The model under review builds one solid part; all positions refer to its coordinate system, in mm. Face numbers are marked on the shaded views. A direction names the side the tool comes from. Round coordinates to 2 decimals unless told otherwise and drop trailing zeros. Loops run counter-clockwise (first coordinate to the right, second up) from the corner with the lowest first, then second, coordinate; pieces in that order, holes last. Notation, with made-up numbers: (-16.75, 5.5) -> (28.25, 5.5) arc R31 cw to (28.25, 42.5) -> close; hole circle Ø10 at (25, -40). An arc over 180 degrees is marked (long way). Write each question's results on one line, items separated by ' | '. Start each with the question number.
Item 1: We need section D-D (z = -7.25). Give the boundary of the cut face in (x, y).
Item 2: Tool access review of the marked faces 1 and 2: name each direction out of +Z, -Z, +X, -X, +Y, -Y from which nothing blocks a thin tool from reaching the whole face with its end or side.
Item 3: We need section B-B (x = -30). Give the boundary of the cut face in (y, z), and give its area (3 significant figures).
Item 4: For L1, parallel to Y at x = 30, z = 13; L2, parallel to Y at x = 60, z = 4.5; L3, parallel to Y at x = 38, z = 10.25, list the stretches that pass through material, from the lowest coordinate up. Write a range as from..to.
Item 5: We need section C-C (x = 9.5). Give the boundary of the cut face in (y, z).
Item 6: Clearance check with flat-ended pins moving along their axes: pin 1 Ø6 at (y, z) = (0, -4) entering from +X; pin 2 Ø5.5 at (x, y) = (-59, -1) entering from +Z; pin 3 Ø1.5 at (y, z) = (3, -1.5) entering from -X. State where each tip first meets the part, or that it passes through.
Item 7: We need section A-A (z = 8.5). Give the boundary of the cut face in (x, y), and give its area (3 significant figures).
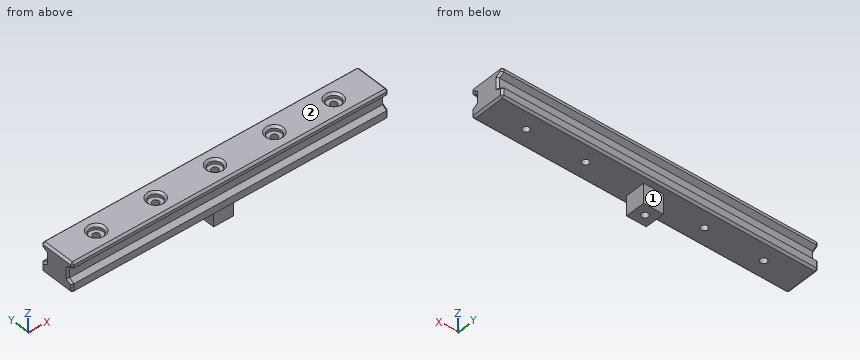
from build123d import *

# Parameters (mm, degrees)
SKETCH1_W                                = 160
SKETCH1_H                                = 18
BOSS_EXTRUDE1_DEPTH                      = 15
CUT_EXTRUDE1_DEPTH                       = 161.953409408
SKETCH3_W                                = 10
SKETCH3_H                                = 10
BOSS_EXTRUDE2_DEPTH                      = 10
CBORE_FOR_M3_PAN_HEAD_SCREW1_D           = 3.4
CBORE_FOR_M3_PAN_HEAD_SCREW1_CBORE_D     = 7
CBORE_FOR_M3_PAN_HEAD_SCREW1_CBORE_DEPTH = 2.4
CHAMFER1_SIZE                            = 1
LPATTERN2_COUNT                          = 3
LPATTERN2_PITCH                          = 30
LPATTERN3_COUNT                          = 3
LPATTERN3_PITCH                          = 30
CHAMFER2_SIZE                            = 1


with BuildPart() as part:
    # Sketch1 → Boss-Extrude1 (new body)
    with BuildSketch(Plane.XY):
        Rectangle(SKETCH1_W, SKETCH1_H)
    extrude(amount=BOSS_EXTRUDE1_DEPTH)

    # Sketch2 → Cut-Extrude1 (cut, through all)
    with BuildSketch(Plane(origin=(80, 0, 0), x_dir=(0, 0, -1), z_dir=(1, 0, 0))):
        Polygon((-12.5, 9), (-4.613248654, 9), (-6.056624327, 6.5), (-11.056624327, 6.5), align=None)
        Polygon((-11.056624327, -6.5), (-12.5, -9), (-4.613248654, -9), (-6.056624327, -6.5), align=None)
    extrude(amount=-CUT_EXTRUDE1_DEPTH, mode=Mode.SUBTRACT)

    # Sketch3 → Boss-Extrude2 (add)
    with BuildSketch(Plane(origin=(0, 0, 0), x_dir=(-1, 0, 0), z_dir=(0, 0, -1))):
        Rectangle(SKETCH3_W, SKETCH3_H)
    extrude(amount=BOSS_EXTRUDE2_DEPTH)

    # CBORE for M3 Pan Head Screw1 (through all)
    with Locations(Plane.XY.offset(15)):
        with Locations((0, 0)):
            cbore_for_m3_pan_head_screw1 = CounterBoreHole(CBORE_FOR_M3_PAN_HEAD_SCREW1_D / 2, CBORE_FOR_M3_PAN_HEAD_SCREW1_CBORE_D / 2, CBORE_FOR_M3_PAN_HEAD_SCREW1_CBORE_DEPTH)

    # Chamfer1
    chamfer1_edges = [part.edges().sort_by_distance(p)[0] for p in [
        (-80, 0, 15),
        (0, -9, 15),
        (80, -9, 2.306624327),
        (-80, -9, 2.306624327),
        (-80, 9, 2.306624327),
        (80, 9, 2.306624327),
        (-80, 7.75, 11.778312164),
        (-80, 7.75, 5.334936491),
        (-80, 6.5, 8.556624327),
        (80, 7.75, 11.778312164),
        (80, 6.5, 8.556624327),
        (80, 7.75, 5.334936491),
        (-80, -6.5, 8.556624327),
        (-80, -7.75, 5.334936491),
        (-80, -7.75, 11.778312164),
        (80, -6.5, 8.556624327),
        (80, -7.75, 11.778312164),
        (80, -7.75, 5.334936491),
        (80, 0, 15),
        (0, -9, 0),
        (-80, 0, 0),
        (0, 9, 0),
        (80, 0, 0),
        (-3.5, 0, 15),
        (0, 9, 15),
        (80, -9, 13.75),
        (-80, -9, 13.75),
        (-80, 9, 13.75),
        (80, 9, 13.75),
    ]]
    chamfer(chamfer1_edges, length=CHAMFER1_SIZE)

    # LPattern2: CBORE for M3 Pan Head Screw1 ×3
    with Locations(*[(i * LPATTERN2_PITCH, 0, 0) for i in range(1, LPATTERN2_COUNT)]):
        add(cbore_for_m3_pan_head_screw1, mode=Mode.SUBTRACT)

    # LPattern3: CBORE for M3 Pan Head Screw1 ×3
    with Locations(*[(-i * LPATTERN3_PITCH, 0, 0) for i in range(1, LPATTERN3_COUNT)]):
        add(cbore_for_m3_pan_head_screw1, mode=Mode.SUBTRACT)

    # Chamfer2
    chamfer2_edges = [part.edges().sort_by_distance(p)[0] for p in [
        (26.5, 0, 15),
        (56.5, 0, 15),
        (-33.5, 0, 15),
        (-63.5, 0, 15),
    ]]
    chamfer(chamfer2_edges, length=CHAMFER2_SIZE)


solid = part.part
Here are the results:
1) outline: (-5, -5) -> (5, -5) -> (5, 5) -> (-5, 5) -> close; hole circle Ø3.4 at (0, 0)
2) face 1: -Z, +X, -X, +Y | face 2: +Z, +X, -X, +Y, -Y
3) outline: (-9, 1) -> (-8, 0) -> (-1.7, 0) -> (-1.7, 12.6) -> (-3.5, 12.6) -> (-3.5, 14) -> (-4.5, 15) -> (-8, 15) -> (-9, 14) -> (-9, 12.5) -> (-6.5, 11.06) -> (-6.5, 6.06) -> (-9, 4.61) -> close; (1.7, 0) -> (8, 0) -> (9, 1) -> (9, 4.61) -> (6.5, 6.06) -> (6.5, 11.06) -> (9, 12.5) -> (9, 14) -> (8, 15) -> (4.5, 15) -> (3.5, 14) -> (3.5, 12.6) -> (1.7, 12.6) -> close | area: 175 mm2
4) L1: y = -9..-3.5, 3.5..9 | L2: y = -9..-1.7, 1.7..9 | L3: y = -6.5..6.5
5) outline: (-9, 1) -> (-8, 0) -> (8, 0) -> (9, 1) -> (9, 4.61) -> (6.5, 6.06) -> (6.5, 11.06) -> (9, 12.5) -> (9, 14) -> (8, 15) -> (-8, 15) -> (-9, 14) -> (-9, 12.5) -> (-6.5, 11.06) -> (-6.5, 6.06) -> (-9, 4.61) -> close
6) pin 1: stops at x = 5 | pin 2: stops at z = 14.66 | pin 3: stops at x = -5
7) outline: (-80, -5.5) -> (-79, -6.5) -> (79, -6.5) -> (80, -5.5) -> (80, 5.5) -> (79, 6.5) -> (-79, 6.5) -> (-80, 5.5) -> close; hole circle Ø3.4 at (-60, 0); hole circle Ø3.4 at (-30, 0); hole circle Ø3.4 at (0, 0); hole circle Ø3.4 at (30, 0); hole circle Ø3.4 at (60, 0) | area: 2,030 mm2
